Geometry check sheet. Reference: the model listing, model coordinates, mm. A direction names the side the tool comes from. Coordinates: 2 decimals unless noted, no trailing zeros. Write each loop counter-clockwise with the first axis right and the second up, starting at its lowest first coordinate (ties: lowest second). Pieces come first, ordered by that corner, then holes. Notation, with made-up numbers: (-7, 17.25) -> (6, 17.25) arc R19 ccw to (6, 39.25) -> close; hole circle Ø7 at (-17, -13). An arc over 180 degrees is marked (long way). Use a Markdown table: item, result.
```python
from build123d import *

# Parameters (mm, degrees)
SKETCH1_R                = 10.668
SKETCH1_R_2              = 7.8994
BOSS_EXTRUDE1_DEPTH      = 69
BOSS_EXTRUDE1_DEPTH_BACK = 69
SKETCH2_R                = 15.23227921
SKETCH2_R_2              = 9.525
CUT_EXTRUDE1_DEPTH       = 12.7
SKETCH3_R                = 15.23227921
SKETCH3_R_2              = 9.525
CUT_EXTRUDE2_DEPTH       = 12.7
CHAMFER1_SIZE            = 0.7874


with BuildPart() as part:
    # Sketch1 → Boss-Extrude1 (new body, two sides)
    with BuildSketch(Plane.XY) as boss_extrude1_sk:
        Circle(SKETCH1_R)
        Circle(SKETCH1_R_2, mode=Mode.SUBTRACT)
    extrude(amount=BOSS_EXTRUDE1_DEPTH)
    extrude(boss_extrude1_sk.sketch, amount=-BOSS_EXTRUDE1_DEPTH_BACK)

    # Sketch2 → Cut-Extrude1 (cut)
    with BuildSketch(Plane.XY.offset(69)):
        Circle(SKETCH2_R)
        Circle(SKETCH2_R_2, mode=Mode.SUBTRACT)
    extrude(amount=-CUT_EXTRUDE1_DEPTH, mode=Mode.SUBTRACT)

    # Sketch3 → Cut-Extrude2 (cut)
    with BuildSketch(Plane(origin=(0, 0, -69), x_dir=(-1, 0, 0), z_dir=(0, 0, -1))):
        Circle(SKETCH3_R)
        Circle(SKETCH3_R_2, mode=Mode.SUBTRACT)
    extrude(amount=-CUT_EXTRUDE2_DEPTH, mode=Mode.SUBTRACT)

    # Chamfer1
    chamfer1_edges = [part.edges().sort_by_distance(p)[0] for p in [
        (-9.525, 0, 69),
        (9.525, 0, -69),
    ]]
    chamfer(chamfer1_edges, length=CHAMFER1_SIZE)


solid = part.part
```
Item 1: Thickness scan on L1, parallel to Y at x = 0, z = 18; L2, parallel to Z at x = -8.5, y = 4.75; L3, parallel to Y at x = -4, z = 42. Record the ranges inside material, lowest first. Write a range as [from, to].
Answer block:
| item | result |
|---|---|
| L1 | y = [-10.67, -7.9], [7.9, 10.67] |
| L2 | z = [-56.3, 56.3] |
| L3 | y = [-9.89, -6.81], [6.81, 9.89] |
Item 2: Tool access check on faces 1 (the cylindrical face through (-7.559, -5.796, 62.34)), 2 (the cylindrical face through (7.559, -5.796, -62.34)), 3 (the cylindrical face through (4.923, -9.464, 0.788)). Record the directions out of +Z, -Z, +X, -X, +Y, -Y that give a thin tool (end or side, any length) a straight path to the whole face; none if there is none.
Answer block:
| item | result |
|---|---|
| face 1 | +Z |
| face 2 | -Z |
| face 3 | +Z, -Z |
Item 3: Depth check by flat-ended pin: P1, Ø1.5, axis at x = -2.5, z = -30.5, coming from the -Y side; P2, Ø6, axis at x = -1, y = 7, coming from the -Z side; P3, Ø8, axis at x = -4.5, z = 35.5, coming from the +Y side; P4, Ø12, axis at x = 7, z = 13.5, coming from the +Y side. Enter the tip coordinate at first touch or a pass-through.
Answer block:
| item | result |
|---|---|
| P1 | stops at y = -10.52 |
| P2 | stops at z = -69 |
| P3 | stops at y = 10.66 |
| P4 | stops at y = 10.62 |
Item 4: Section check A-A on x = 0. Record the boundary of the cut face in (y, z) (3 decimals).
Answer block:
| item | result |
|---|---|
| outline | (-10.668, -56.3) -> (-9.525, -56.3) -> (-9.525, -68.213) -> (-8.738, -69) -> (-7.899, -69) -> (-7.899, 69) -> (-8.738, 69) -> (-9.525, 68.213) -> (-9.525, 56.3) -> (-10.668, 56.3) -> close; (7.899, -69) -> (8.738, -69) -> (9.525, -68.213) -> (9.525, -56.3) -> (10.668, -56.3) -> (10.668, 56.3) -> (9.525, 56.3) -> (9.525, 68.213) -> (8.738, 69) -> (7.899, 69) -> close |
Item 5: Section check C-C on z = -47. Record the boundary of the cut face in (x, y), then the cut area to 3 significant figures.
Answer block:
| item | result |
|---|---|
| outline | circle Ø21.34 at (0, 0); hole circle Ø15.8 at (0, 0) |
| area | 161 mm^2 |
